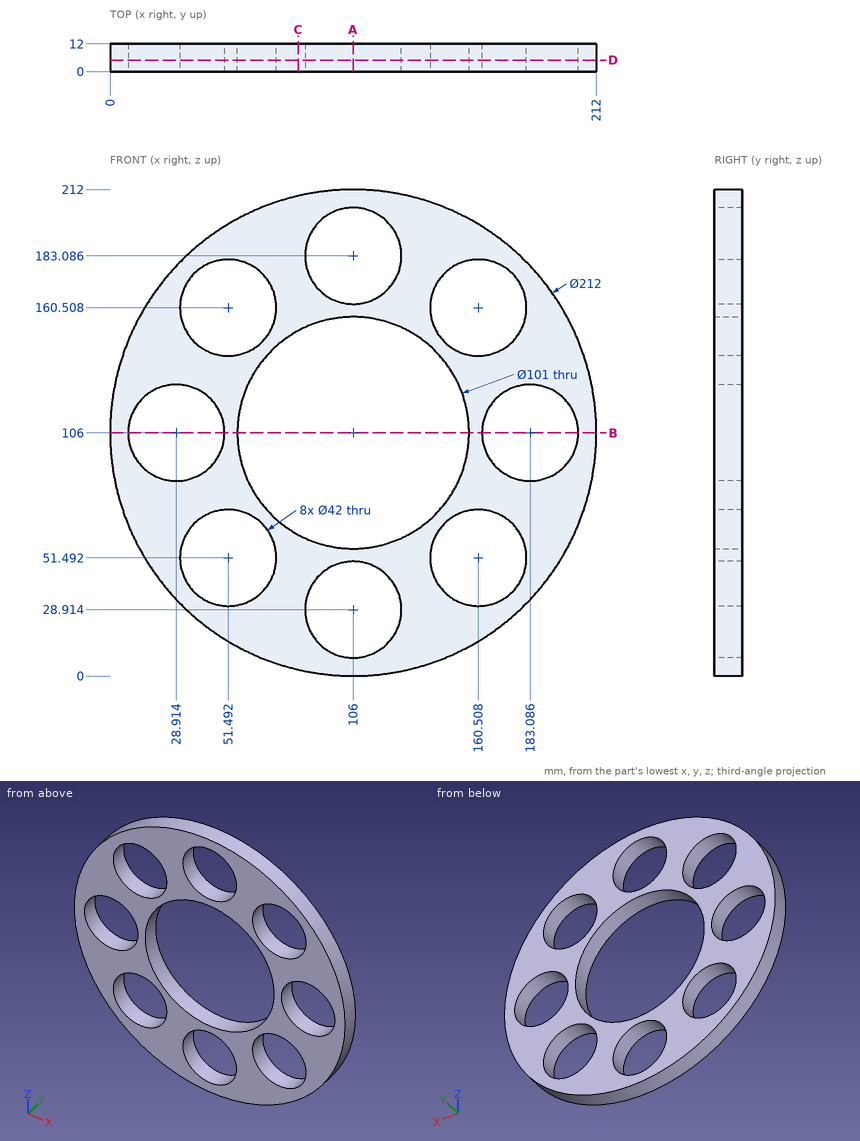
Check sheet for the drawn part. Datum: minimum x, y, z corner. Units: mm. Round coordinates to 2 decimals unless told otherwise and drop trailing zeros. Order: outer loops, then holes, each group sorted by start corner. A loop starts at its lowest first (then second) coordinate and runs counter-clockwise, first axis right, second up. Notation, with made-up numbers: (48.5, 12.5) -> (100.5, 12.5) arc R20 ccw to (100.5, 33.5) -> close; hole circle Ø5 at (16, -31.75). An arc over 180 degrees is marked (long way). Put each result on its own line as item: value. Start each with the question number.
(1) Section check D-D (y = 5). State how many separate pieces and enclosed holes the cut face has, then the cut area to 3 significant figures.
(2) Depth check by flat-ended pin: pin 1 Ø25 at (x, z) = (160.51, 160.51) entering from -Y; pin 2 Ø4 at (y, z) = (11, 48) entering from -X; pin 3 Ø6 at (y, z) = (3, 164.5) entering from -X; pin 4 Ø1 at (x, y) = (43, 7.5) entering from +Z. Enter the tip coordinate at first touch or a pass-through.
(3) Material ranges on line 1 along X through (y, z) = (11.25, 105); line 2 along Z through (x, y) = (98.5, 10.5); line 3 along Z through (x, y) = (64.5, 9.5) (1 decimal), recorded low to high.
(4) Section check B-B (z = 106). Enter the section's corners in (x, y).
(5) Section check A-A (x = 106). Enter the section's corners in (y, z).
(6) Section check C-C (x = 82). Enter the section's corners in (y, z), then the cut area to 3 significant figures.
Completed:
1. separate pieces: 1
1. enclosed holes: 9
1. area: 16,200 mm2
2. pin 1: passes through
2. pin 2: stops at x = 16
2. pin 3: stops at x = 15.69
2. pin 4: stops at z = 191.61
3. line 1: x = 0 to 7.94, 49.89 to 55.51, 156.49 to 162.11, 204.06 to 212
3. line 2: z = 0.27 to 9.3, 48.53 to 56.06, 155.94 to 163.47, 202.7 to 211.73
3. line 3: z = 8.5 to 35, 68 to 77.2, 134.8 to 144, 177 to 203.5
4. outline: (0, 0) -> (7.91, 0) -> (7.91, 12) -> (0, 12) -> close; (49.91, 0) -> (55.5, 0) -> (55.5, 12) -> (49.91, 12) -> close; (156.5, 0) -> (162.09, 0) -> (162.09, 12) -> (156.5, 12) -> close; (204.09, 0) -> (212, 0) -> (212, 12) -> (204.09, 12) -> close
5. outline: (0, 0) -> (12, 0) -> (12, 7.91) -> (0, 7.91) -> close; (0, 49.91) -> (12, 49.91) -> (12, 55.5) -> (0, 55.5) -> close; (0, 156.5) -> (12, 156.5) -> (12, 162.09) -> (0, 162.09) -> close; (0, 204.09) -> (12, 204.09) -> (12, 212) -> (0, 212) -> close
6. outline: (0, 2.75) -> (12, 2.75) -> (12, 61.57) -> (0, 61.57) -> close; (0, 150.43) -> (12, 150.43) -> (12, 209.25) -> (0, 209.25) -> close
6. area: 1,410 mm2
